```python
from build123d import *

# Parameters (mm, degrees)
SKETCH1_R           = 12.7
BOSS_EXTRUDE1_DEPTH = 2.286
SKETCH2_R           = 1.6002
CUT_EXTRUDE1_DEPTH  = 3.286
CIRPATTERN1_COUNT   = 4
SKETCH4_R           = 1.6002
BOSS_EXTRUDE3_DEPTH = 0.762
CHAMFER1_SIZE       = 0.635
SKETCH5_R           = 3.0861
BOSS_EXTRUDE4_DEPTH = 0.9525
CHAMFER2_SIZE       = 0.635


with BuildPart() as part:
    # Sketch1 → Boss-Extrude1 (new body)
    with BuildSketch(Plane(origin=(0, 0, 0), x_dir=(1, 0, 0), z_dir=(0, 1, 0))):
        Circle(SKETCH1_R)
        with BuildLine():
            Line((-1.1176, 0.998384796), (1.1176, 0.998384796))
            ThreePointArc((1.1176, 0.998384796), (0, -1.4986), (-1.1176, 0.998384796))
        make_face(mode=Mode.SUBTRACT)
    extrude(amount=BOSS_EXTRUDE1_DEPTH)

    # Sketch2 → Cut-Extrude1 (cut, through all)
    with BuildSketch(Plane(origin=(0, 2.286, 0), x_dir=(1, 0, 0), z_dir=(0, 1, 0))):
        with Locations((-10.31875, 0)):
            Circle(SKETCH2_R)
    cut_extrude1 = extrude(amount=-CUT_EXTRUDE1_DEPTH, mode=Mode.SUBTRACT)

    # CirPattern1: Cut-Extrude1 ×4 about axis
    cirpattern1_axis = Axis((0, 0, 0), (0, 1, 0))
    for i in range(1, CIRPATTERN1_COUNT):
        add(cut_extrude1.rotate(cirpattern1_axis, i * 360 / CIRPATTERN1_COUNT), mode=Mode.SUBTRACT)

    # Sketch4 → Boss-Extrude3 (add)
    with BuildSketch(Plane(origin=(0, 2.286, 0), x_dir=(1, 0, 0), z_dir=(0, 1, 0))):
        with BuildLine():
            ThreePointArc((-12.242958262, -3.376384606), (-6.43255, 0), (-12.242958262, 3.376384606))
            ThreePointArc((-12.242958262, 3.376384606), (-12.7, 0), (-12.242958262, -3.376384606))
        make_face()
        with Locations((-10.31875, 0)):
            Circle(SKETCH4_R, mode=Mode.SUBTRACT)
        with BuildLine():
            ThreePointArc((-3.376384606, 12.242958262), (0, 6.43255), (3.376384606, 12.242958262))
            ThreePointArc((3.376384606, 12.242958262), (0, 12.7), (-3.376384606, 12.242958262))
        make_face()
        with Locations((0, 10.31875)):
            Circle(SKETCH4_R, mode=Mode.SUBTRACT)
        with BuildLine():
            ThreePointArc((12.242958262, 3.376384606), (6.43255, 0), (12.242958262, -3.376384606))
            ThreePointArc((12.242958262, -3.376384606), (12.7, 0), (12.242958262, 3.376384606))
        make_face()
        with Locations((10.31875, 0)):
            Circle(SKETCH4_R, mode=Mode.SUBTRACT)
        with BuildLine():
            ThreePointArc((3.376384606, -12.242958262), (0, -6.43255), (-3.376384606, -12.242958262))
            ThreePointArc((-3.376384606, -12.242958262), (0, -12.7), (3.376384606, -12.242958262))
        make_face()
        with Locations((0, -10.31875)):
            Circle(SKETCH4_R, mode=Mode.SUBTRACT)
    extrude(amount=BOSS_EXTRUDE3_DEPTH)

    # Chamfer1
    chamfer1_edges = [part.edges().sort_by_distance(p)[0] for p in [
        (-1.6002, 3.048, -10.31875),
        (8.71855, 3.048, 0),
        (-11.91895, 3.048, 0),
        (-1.6002, 3.048, 10.31875),
    ]]
    chamfer(chamfer1_edges, length=CHAMFER1_SIZE)

    # Sketch5 → Boss-Extrude4 (add)
    with BuildSketch(Plane.XZ):
        Circle(SKETCH5_R)
        with BuildLine():
            Line((1.1176, -0.998384796), (-1.1176, -0.998384796))
            ThreePointArc((-1.1176, -0.998384796), (0, 1.4986), (1.1176, -0.998384796))
        make_face(mode=Mode.SUBTRACT)
    extrude(amount=BOSS_EXTRUDE4_DEPTH)

    # Chamfer2
    chamfer2_edges = [part.edges().sort_by_distance(p)[0] for p in [
        (-3.0861, -0.9525, 0),
    ]]
    chamfer(chamfer2_edges, length=CHAMFER2_SIZE)


solid = part.part
```
Verification items for the finished model (mm, model axes). A direction names the side the tool comes from. Coordinates: 2 decimals unless noted, no trailing zeros. Loops run counter-clockwise (first coordinate to the right, second up) from the corner with the lowest first, then second, coordinate; pieces in that order, holes last. Notation, with made-up numbers: (55.25, 76) -> (65.25, 76) arc R24 cw to (65.25, 103) -> close; hole circle Ø10 at (-27, -23.5). An arc over 180 degrees is marked (long way). Answer in a Markdown table with one row per item. Add a question column.
1. Section check A-A, the plane x = 0. Give the number of separate pieces and of enclosed holes in the cut face, then the cut area to 3 significant figures.
2. Section check B-B, the plane y = 0.9. Enter the section's corners in (x, z), then the cut area to 3 significant figures.
3. Draft check along Z on faces 4 (the face through (0, -0.952, -2)), 5 (the face through (6.434, 2.662, -0.114)), 6 (the face through (0.114, 2.662, 6.434)). Enter one of: +Z half, -Z half, draft (parallel to the pull), parting line (faces both ways), or undercut.
4. Access from +Z, -Z, +X, -X, +Y, -Y to the whole of each face (thin tool, end or side, straight path). Record for faces 1 (the face through (0, 2.286, 3)), 2 (the face through (-2.449, -0.157, -1.878)), 3 (the face through (-8, 3.048, -1)).
5. Material ranges on probe 1 along X at (y, z) = (0.4, 1); probe 2 along Z at (x, y) = (-0.75, 2.35); probe 3 along Y at (x, z) = (-0.75, -5), recorded low to high. Write a range as [from, to].
6. Depth check by flat-ended pin: P1, Ø12, axis at x = 9, z = 9.5, coming from the -Y side; P2, Ø3.5, axis at x = 0, z = 0, coming from the +Y side; P3, Ø0.5, axis at x = -0.5, y = -0.5, coming from the +Z side. Enter the tip coordinate at first touch or a pass-through.
Derived:
| question | item | result |
|---|---|---|
| 1 | separate pieces | 4 |
| 1 | enclosed holes | 0 |
| 1 | area | 44.7 mm² |
| 2 | outline | circle Ø25.4 at (0, 0); hole circle Ø3.2 at (-10.32, 0); hole circle Ø3.2 at (0, -10.32); hole circle Ø3.2 at (0, 10.32); hole (-1.12, -1) -> (1.12, -1) arc R1.5 ccw (long way) to start; hole circle Ø3.2 at (10.32, 0) |
| 2 | area | 468 mm² |
| 3 | face 4 | draft |
| 3 | face 5 | parting line |
| 3 | face 6 | undercut |
| 4 | face 1 | +Y |
| 4 | face 2 | -Y |
| 4 | face 3 | +Z, -Z, +X, -X, +Y |
| 5 | probe 1 | x = [-12.66, -11.57], [-9.07, -1.12], [1.12, 9.07], [11.57, 12.66] |
| 5 | probe 2 | z = [-12.68, -11.73], [-8.91, -6.51], [6.51, 8.91], [11.73, 12.68] |
| 5 | probe 3 | y = [0, 2.29] |
| 6 | P1 | stops at y = 0 |
| 6 | P2 | stops at y = 2.29 |
| 6 | P3 | stops at z = 3.07 |
